Check sheet for the modelled part. Datum: model origin and axes. Units: mm. Face numbers are marked on the shaded views. Coordinates: 2 decimals unless noted, no trailing zeros. Loops run counter-clockwise (first coordinate to the right, second up) from the corner with the lowest first, then second, coordinate; pieces in that order, holes last. Notation, with made-up numbers: (-6, 32) -> (51, 32) arc R12 ccw to (51, 44) -> close; hole circle Ø1 at (6.25, -14.75). An arc over 180 degrees is marked (long way). Use one line per item in the form item = value.
from build123d import *

# Parameters (mm, degrees)
PAD_DEPTH    = 15
POCKET_DEPTH = 13
PAD001_DEPTH = 55


with BuildPart() as part:
    # Sketch → Pad (new body)
    with BuildSketch(Plane.XZ):
        with BuildLine():
            ThreePointArc((8.889624, 1.945402), (-9.099882, -0.046426), (8.90901, -1.854598))
            Line((10.40901, -1.854598), (8.90901, -1.854598))
            Line((10.40901, 1.945402), (10.40901, -1.854598))
            Line((8.889624, 1.945402), (10.40901, 1.945402))
        make_face()
    extrude(amount=PAD_DEPTH)

    # Sketch001 (on Face6 of Pad) → Pocket (cut)
    with BuildSketch(Plane.XZ.offset(15)):
        Polygon((-1.5, 7), (1.5, 7), (1.5, -7), (-3.348355, -7), (-3.348355, -3.808815), (-1.5, -3.808815), align=None)
    extrude(amount=-POCKET_DEPTH, mode=Mode.SUBTRACT)

    # Sketch002 (on Face5 of Pocket) → Pad001 (join)
    with BuildSketch(Plane.XZ.offset(15)):
        with BuildLine():
            Line((0, 7), (-1.5, 7))
            Line((-1.5, 7), (-1.5, -3.808815))
            Line((-1.5, -3.808815), (-3.348355, -3.808815))
            Line((-3.348355, -3.808815), (-3.348355, -7))
            Line((-3.348355, -7), (0, -7))
            Line((0, -7), (0, -9.054887))
            ThreePointArc((0, 9.054887), (-9.054887, 0), (0, -9.054887))
            Line((0, 7), (0, 9.054887))
        make_face()
    extrude(amount=PAD001_DEPTH)


solid = part.part
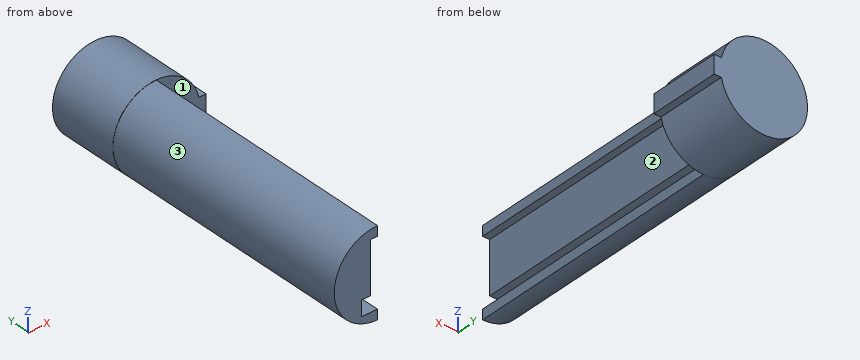
(1) Section check D-D, the plane x = -7.5. Record the boundary of the cut face in (y, z).
Established:
outline = (-70, -5.07) -> (-15, -5.07) -> (-15, -5.15) -> (0, -5.15) -> (0, 5.15) -> (-15, 5.15) -> (-15, 5.07) -> (-70, 5.07) -> close
(2) Section check B-B, the plane z = 0. Record the boundary of the cut face in (x, y).
Established:
outline = (-9.1, -15) -> (-9.05, -15) -> (-9.05, -70) -> (-1.5, -70) -> (-1.5, -2) -> (1.5, -2) -> (1.5, -15) -> (10.41, -15) -> (10.41, 0) -> (-9.1, 0) -> close
(3) Scan lines: line 1 along Z through (x, y) = (0.25, -10); line 2 along Y through (x, z) = (4.25, -2.75); line 3 along Y through (x, z) = (1.25, -1.25). Record each from-to range of solid material in increasing order.
Established:
line_1 = -9.1 to -7, 7 to 9.1
line_2 = -15 to 0
line_3 = -2 to 0
(4) Go/stop test with flat-tipped pins: P1, Ø2.5, axis at y = -47.5, z = -5, coming from the +X side; P2, Ø0.8, axis at x = 9.5, y = -4, coming from the -Z side; P3, Ø5.5, axis at x = 1.5, z = -1.5, coming from the -Y side. Record where each tip stops, or that it passes through.
Established:
P1 = -1.5
P2 = -1.85
P3 = -15
(5) Section check C-C, the plane y = -27. Record the boundary of the cut face in (x, z), plus the area to 3 significant figures.
Established:
outline = (-3.35, -7) -> (-3.35, -3.81) -> (-1.5, -3.81) -> (-1.5, 7) -> (0, 7) -> (0, 9.05) arc R9.05 ccw to (0, -9.05) -> (0, -7) -> close
area = 102 mm²
(6) Mould release check, pull along Z, two halves, no side actions. Record for the marked faces 1, 2 and 3: +Z half, -Z half, draft (parallel to the pull), parting line (faces both ways), or undercut.
Established:
face_1 = draft
face_2 = undercut
face_3 = parting line
(7) Section check A-A, the plane y = -9. Record the boundary of the cut face in (x, z).
Established:
outline = (8.89, 1.95) arc R9.1 ccw (long way) to (8.91, -1.85) -> (10.41, -1.85) -> (10.41, 1.95) -> close; hole (-3.35, -7) -> (1.5, -7) -> (1.5, 7) -> (-1.5, 7) -> (-1.5, -3.81) -> (-3.35, -3.81) -> close
